Source: CAD feature listing. Evaluate the final solid. Frame: model axes, mm. Face numbers are marked on the shaded views. A direction names the side the tool comes from. Give positions to 0.01 mm unless a question says otherwise; leave off trailing zeros. Loops run counter-clockwise (first coordinate to the right, second up) from the corner with the lowest first, then second, coordinate; pieces in that order, holes last. Notation, with made-up numbers: M 84,-15 L 88,-15 A15 cw 88,-8 Z; hole C 3,-10.75 d2. An arc over 180 degrees is marked long. Answer in a Markdown table with one row per item.
```python
from build123d import *

# Parameters (mm, degrees)
F0_W     = 400
F0_H     = 300
F0_W_2   = 390.000014
F0_H_2   = 290.000014
F1_DEPTH = 150
F2_W     = 390.000014
F2_H     = 290.000014
F3_DEPTH = 1


with BuildPart() as f1:
    # F0 (on Front) → F1 (new body)
    with BuildSketch(Plane.XZ):
        Rectangle(F0_W, F0_H)
        Rectangle(F0_W_2, F0_H_2, mode=Mode.SUBTRACT)
    extrude(amount=F1_DEPTH)

    # F2 (on face) → F3 (join)
    with BuildSketch(Plane(origin=(0, 0, 0), x_dir=(-1, 0, 0), z_dir=(0, 1, 0))):
        Rectangle(F2_W, F2_H)
    extrude(amount=-F3_DEPTH)


solid = f1.part
```
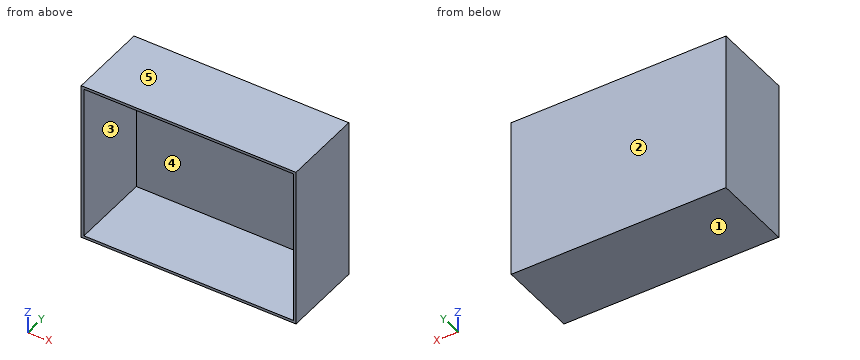
1) Section A-A, the plane y = -95.5. Return loops of the section in (x, z), then the cut area to 3 significant figures.
Reply:
| item | result |
|---|---|
| outline | M -200,-150 L 200,-150 L 200,150 L -200,150 Z; hole M -195,-145 L 195,-145 L 195,145 L -195,145 Z |
| area | 6,900 mm² |
2) Pin query (flat end, axial travel): pin 1 Ø2 at (x, z) = (121, 31.5) entering from +Y; pin 2 Ø2 at (x, z) = (-67.5, 66) entering from -Y. Return the tip coordinate at first contact, or that it passes through.
Reply:
| item | result |
|---|---|
| pin 1 | stops at y = 0 |
| pin 2 | stops at y = -1 |
3) Pull-direction query (Z, two-part tool) for the marked faces 1, 2 and 3; classes: released by +Z, released by -Z, zero draft, split by the parting line, or undercut.
Reply:
| item | result |
|---|---|
| face 1 | released by -Z |
| face 2 | zero draft |
| face 3 | undercut |
4) Material intervals for L1, parallel to Z at x = -20, y = -90; L2, parallel to X at y = -82.5, z = 99.5; L3, parallel to Y at x = 8.5, z = -75.5, sorted ascending.
Reply:
| item | result |
|---|---|
| L1 | z = -150 to -145, 145 to 150 |
| L2 | x = -200 to -195, 195 to 200 |
| L3 | y = -1 to 0 |
5) Set-up query: the marked faces 4 and 5. Return all of +Z, -Z, +X, -X, +Y, -Y with unobstructed straight access to the full face (end or side cutting, diameter ignored); none if empty.
Reply:
| item | result |
|---|---|
| face 4 | -Y |
| face 5 | +Z, +X, -X, +Y, -Y |
6) Section C-C, the plane x = -162.5. Return loops of the section in (y, z), then the cut area to 3 significant figures.
Reply:
| item | result |
|---|---|
| outline | M -150,-150 L 0,-150 L 0,150 L -150,150 L -150,145 L -1,145 L -1,-145 L -150,-145 Z |
| area | 1,790 mm² |
7) Section B-B, the plane z = 43.5. Return loops of the section in (x, y).
Reply:
| item | result |
|---|---|
| outline | M -200,-150 L -195,-150 L -195,-1 L 195,-1 L 195,-150 L 200,-150 L 200,0 L -200,0 Z |
